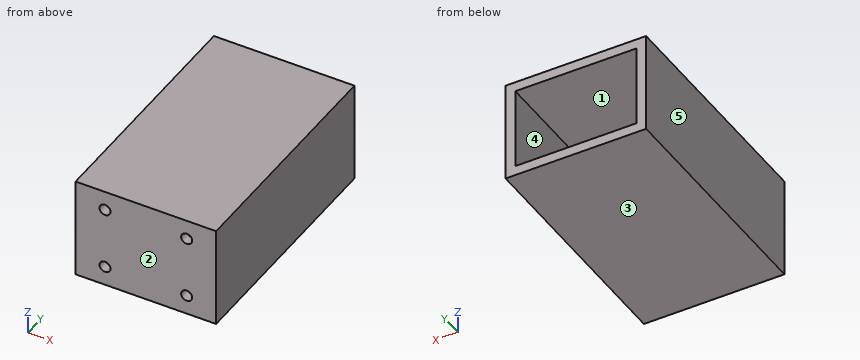
from build123d import *

# Parameters (mm, degrees)
SKETCH1_W            = 43
SKETCH1_H            = 31
BOSS_EXTRUDE1_DEPTH  = 3
BOSS_EXTRUDE2_START  = 3
SKETCH1_3_W          = 43
SKETCH1_3_H          = 31
SKETCH1_3_W_2        = 37
SKETCH1_3_H_2        = 25
BOSS_EXTRUDE2_DEPTH  = 70
M3_CLEARANCE_HOLE1_D = 3.4


with BuildPart() as part:
    # Sketch1 → Boss-Extrude1 (new body)
    with BuildSketch(Plane(origin=(0, 0, 0), x_dir=(1, 0, 0), z_dir=(0, 1, 0))):
        Rectangle(SKETCH1_W, SKETCH1_H)
    extrude(amount=BOSS_EXTRUDE1_DEPTH)

    # Sketch1<3> → Boss-Extrude2 (add)
    with BuildSketch(Plane(origin=(0, 0, 0), x_dir=(1, 0, 0), z_dir=(0, 1, 0)).offset(BOSS_EXTRUDE2_START)):
        Rectangle(SKETCH1_3_W, SKETCH1_3_H)
        Rectangle(SKETCH1_3_W_2, SKETCH1_3_H_2, mode=Mode.SUBTRACT)
    extrude(amount=BOSS_EXTRUDE2_DEPTH)

    # M3 Clearance Hole1 (through all)
    with Locations(Plane(origin=(0, 3, 0), x_dir=(1, 0, 0), z_dir=(0, 1, 0))):
        with Locations((-12.5, 9.5), (12.5, 9.5), (12.5, -9.5), (-12.5, -9.5)):
            Hole(M3_CLEARANCE_HOLE1_D / 2)


solid = part.part
Source: CAD feature listing. Evaluate the final solid. Frame: model axes, mm. Face numbers are marked on the shaded views. A direction names the side the tool comes from. Give positions to 0.01 mm unless a question says otherwise; leave off trailing zeros. Write each loop counter-clockwise with the first axis right and the second up, starting at its lowest first coordinate (ties: lowest second). Pieces come first, ordered by that corner, then holes. Notation, with made-up numbers: (86.25, 41) -> (144.25, 41) arc R30 ccw to (144.25, 79) -> close; hole circle Ø11 at (66, 53.5). An arc over 180 degrees is marked (long way). Write item = value, one per line.
Q1. Cut plane A-A on x = 12.5. Return loops of the section in (y, z).
Here are the results:
outline = (0, -15.5) -> (73, -15.5) -> (73, -12.5) -> (3, -12.5) -> (3, -11.2) -> (0, -11.2) -> close; (0, -7.8) -> (3, -7.8) -> (3, 7.8) -> (0, 7.8) -> close; (0, 11.2) -> (3, 11.2) -> (3, 12.5) -> (73, 12.5) -> (73, 15.5) -> (0, 15.5) -> close
Q2. Mould query, pull axis X, two halves, no side actions, for the marked faces 3, 4 and 5. Classes: +X half, -X half, draft (parallel to the pull), parting line (faces both ways), or undercut.
Here are the results:
face_3 = draft
face_4 = undercut
face_5 = -X half
Q3. Reachability of the marked faces 1 and 2 from +Z, -Z, +X, -X, +Y, -Y: full face, straight path, thin tool, end or side. Return the list, or none.
Here are the results:
face_1 = +Y
face_2 = +Z, -Z, +X, -X, -Y
Q4. Cut plane C-C on z = -9.5. Return loops of the section in (x, y).
Here are the results:
outline = (-21.5, 0) -> (-14.2, 0) -> (-14.2, 3) -> (-18.5, 3) -> (-18.5, 73) -> (-21.5, 73) -> close; (-10.8, 0) -> (10.8, 0) -> (10.8, 3) -> (-10.8, 3) -> close; (14.2, 0) -> (21.5, 0) -> (21.5, 73) -> (18.5, 73) -> (18.5, 3) -> (14.2, 3) -> close
Q5. Cut plane B-B on y = 26. Return loops of the section in (x, z), then the cut area to 3 significant figures.
Here are the results:
outline = (-21.5, -15.5) -> (21.5, -15.5) -> (21.5, 15.5) -> (-21.5, 15.5) -> close; hole (-18.5, -12.5) -> (18.5, -12.5) -> (18.5, 12.5) -> (-18.5, 12.5) -> close
area = 408 mm²
Q6. Line query: line 1 (X direction, y = 1.35, z = 9.5); line 2 (Z direction, x = 12.5, y = 0.8); line 3 (Z direction, x = 13.5, y = 50.5). Output: solid intervals per line, ascending. Write a range as from..to.
Here are the results:
line_1 = -21.5..-14.2, -10.8..10.8, 14.2..21.5
line_2 = -15.5..-11.2, -7.8..7.8, 11.2..15.5
line_3 = -15.5..-12.5, 12.5..15.5
Q7. First-contact query: pin 1 (4.5 mm diameter, centred on x = -12.5, z = 9.5, fed in from +Y); pin 2 (3 mm diameter, centred on x = -12.5, z = -9.5, fed in from -Y). Flat tips, straight axial feed; report the tip coordinate or a pass-through.
Here are the results:
pin_1 = 3
pin_2 = through
Q8. Cut plane D-D on x = -15. Return loops of the section in (y, z).
Here are the results:
outline = (0, -15.5) -> (73, -15.5) -> (73, -12.5) -> (3, -12.5) -> (3, 12.5) -> (73, 12.5) -> (73, 15.5) -> (0, 15.5) -> close
